Design review of the part built by this model. Coordinates are the model's own, in mm. A direction names the side the tool comes from. Round coordinates to 2 decimals unless told otherwise and drop trailing zeros. Write each loop counter-clockwise with the first axis right and the second up, starting at its lowest first coordinate (ties: lowest second). Pieces come first, ordered by that corner, then holes. Notation, with made-up numbers: (15, -20.5) -> (46, -20.5) arc R25 cw to (46, 12.5) -> close; hole circle Ø9 at (46, -2). An arc over 180 degrees is marked (long way). Write item = value, one per line. Start each with the question number.
Item 1: For pin 1 Ø1.2 at (x, y) = (35, 0) entering from +Z; pin 2 Ø1.5 at (y, z) = (2, -10) entering from +X; pin 3 Ø3 at (y, z) = (1, 24) entering from +X; pin 4 Ø2 at (y, z) = (-3, -0.5) entering from +X, all flat-tipped, find the tip position at first contact; note any pin that passes through.
Item 2: Add section A-A, the plane y = -3. State the section outline as (x, z) points.
Item 3: Mouldability with a two-part tool opening along Z and no side actions: class faces 1 (the flat face through (30, 0, 32)), 2 (the flat face through (-25, 0, 0)), 3 (the flat face through (-30, 0, 32)), 4 (the flat face through (-10, 0, -7)) as released by +Z, released by -Z, zero draft, split by the parting line, or undercut.
Item 4: Add section B-B, the plane x = -16. State the section outline as (y, z) points.
Item 5: Machinability: for faces 5 (the flat face through (20, 0, 17)), 6 (the flat face through (-30, 0, 2)), 7 (the cylindrical face through (-40, 0, 33)), 8 (the cylindrical face through (40, 0, 1)), which of the approach directions +Z, -Z, +X, -X, +Y, -Y give a long, thin tool a straight path to every point of the face, cutting with its end or side? Answer none if there is none.
Item 6: Add section C-C, the plane z = 21.5. State the section outline as (x, y) points, then the cut area to 3 significant figures.
Item 7: To check wall thickness, follow L1, parallel to X at y = 0, z = 33.45; L2, parallel to Z at x = 23, y = -3.25; L3, parallel to Y at x = 35, z = -5. State the ranges of each line that lie inside material, in increasing order.
from build123d import *

# Parameters (mm, degrees)
EXTRUDE_1_DEPTH          = 34
SKETCH_2_R               = 1
CUT_EXTRUDE_4_DEPTH      = 35
CUT_EXTRUDE_4_DEPTH_BACK = 30
SKETCH_3_W               = 20
SKETCH_3_H               = 30
CUT_EXTRUDE_5_DEPTH      = 30
CUT_EXTRUDE_5_DEPTH_BACK = 30
EXTRUDE_4_DEPTH          = 15
SKETCH_5_R               = 1
CUT_EXTRUDE_7_DEPTH      = 16
SKETCH_6_W               = 15
SKETCH_6_H               = 10
EXTRUDE_5_DEPTH          = 10


with BuildPart() as part:
    # 草圖1 → 填料-伸長1 (new body)
    with BuildSketch(Plane.XY):
        with BuildLine():
            Line((-35, 5), (35, 5))
            ThreePointArc((35, 5), (40, 0), (35, -5))
            Line((35, -5), (-35, -5))
            ThreePointArc((-35, -5), (-40, 0), (-35, 5))
        make_face()
    extrude(amount=EXTRUDE_1_DEPTH)

    # 草圖2 → 除料-伸長4 (cut, two sides)
    with BuildSketch(Plane.XY) as cut_extrude_4_sk:
        with Locations((-35, 0)):
            Circle(SKETCH_2_R)
        with Locations((35, 0)):
            Circle(SKETCH_2_R)
    extrude(amount=CUT_EXTRUDE_4_DEPTH, mode=Mode.SUBTRACT)
    extrude(cut_extrude_4_sk.sketch, amount=-CUT_EXTRUDE_4_DEPTH_BACK, mode=Mode.SUBTRACT)

    # 草圖3 → 除料-伸長5 (cut, two sides)
    with BuildSketch(Plane(origin=(0, 0, 0), x_dir=(1, 0, 0), z_dir=(0, 1, 0))) as cut_extrude_5_sk:
        with Locations((-30, -17)):
            Rectangle(SKETCH_3_W, SKETCH_3_H)
        with Locations((30, -17)):
            Rectangle(SKETCH_3_W, SKETCH_3_H)
    extrude(amount=CUT_EXTRUDE_5_DEPTH, mode=Mode.SUBTRACT)
    extrude(cut_extrude_5_sk.sketch, amount=-CUT_EXTRUDE_5_DEPTH_BACK, mode=Mode.SUBTRACT)

    # 草圖4 → 填料-伸長4 (add)
    with BuildSketch(Plane.XY):
        with BuildLine():
            Line((0, 5), (105, 5))
            ThreePointArc((105, 5), (110, 0), (105, -5))
            Line((105, -5), (0, -5))
            Line((0, -5), (0, 5))
        make_face()
    extrude(amount=-EXTRUDE_4_DEPTH)

    # 草圖5 → 除料-伸長7 (cut, through all)
    with BuildSketch(Plane.XY):
        with Locations((35, 0)):
            Circle(SKETCH_5_R)
        with Locations((105, 0)):
            Circle(SKETCH_5_R)
    extrude(amount=-CUT_EXTRUDE_7_DEPTH, mode=Mode.SUBTRACT)

    # 草圖6 → 填料-伸長5 (add)
    with BuildSketch(Plane(origin=(0, 0, 0), x_dir=(0, 0, -1), z_dir=(1, 0, 0))):
        with Locations((7.5, 0)):
            Rectangle(SKETCH_6_W, SKETCH_6_H)
    extrude(amount=-EXTRUDE_5_DEPTH)


solid = part.part
Result set:
q1.pin_1 = through
q1.pin_2 = 109.84
q1.pin_3 = 20
q1.pin_4 = 109.58
q2.outline = (-39, 0) -> (-10, 0) -> (-10, -15) -> (109, -15) -> (109, 0) -> (39, 0) -> (39, 2) -> (20, 2) -> (20, 32) -> (39, 32) -> (39, 34) -> (-39, 34) -> (-39, 32) -> (-20, 32) -> (-20, 2) -> (-39, 2) -> close
q3.face_1 = undercut
q3.face_2 = released by -Z
q3.face_3 = undercut
q3.face_4 = zero draft
q4.outline = (-5, 0) -> (5, 0) -> (5, 34) -> (-5, 34) -> close
q5.face_5 = +X, +Y, -Y
q5.face_6 = -X, +Y, -Y
q5.face_7 = +Z, -Z, -X
q5.face_8 = +Z, +X
q6.outline = (-20, -5) -> (20, -5) -> (20, 5) -> (-20, 5) -> close
q6.area = 400 mm²
q7.L1 = -40 to -36, -34 to 34, 36 to 40
q7.L2 = -15 to 2, 32 to 34
q7.L3 = -5 to -1, 1 to 5
